For this review, take the finished solid that the model builds, in its own axes (mm). Face numbers are marked on the shaded views. A direction names the side the tool comes from. Coordinates: 2 decimals unless noted, no trailing zeros. Write each loop counter-clockwise with the first axis right and the second up, starting at its lowest first coordinate (ties: lowest second). Pieces come first, ordered by that corner, then holes. Notation, with made-up numbers: M 73.5,-1 L 87.5,-1 A27 ccw 87.5,26 Z; hole C 42,25 d10. An arc over 180 degrees is marked long. One line per question, with ' | ' between items.
from build123d import *

# Parameters (mm, degrees)
SKETCH1_R           = 6.35
BOSS_EXTRUDE1_DEPTH = 25.4
SKETCH2_W           = 26.416
SKETCH2_H           = 39.116
CUT_EXTRUDE1_DEPTH  = 26.4
SKETCH3_R           = 3.683
CUT_EXTRUDE2_DEPTH  = 6.842


with BuildPart() as part:
    # Sketch1 → Boss-Extrude1 (new body)
    with BuildSketch(Plane.XY):
        with BuildLine():
            Line((-50.8, 12.7), (50.8, 12.7))
            ThreePointArc((50.8, 12.7), (63.5, 0), (50.8, -12.7))
            Line((50.8, -12.7), (-50.8, -12.7))
            ThreePointArc((-50.8, -12.7), (-63.5, 0), (-50.8, 12.7))
        make_face()
        with Locations((-50.8, 0)):
            Circle(SKETCH1_R, mode=Mode.SUBTRACT)
        with Locations((50.8, 0)):
            Circle(SKETCH1_R, mode=Mode.SUBTRACT)
    extrude(amount=BOSS_EXTRUDE1_DEPTH)

    # Sketch2 → Cut-Extrude1 (cut, through all)
    with BuildSketch(Plane(origin=(0, 12.7, 0), x_dir=(1, 0, 0), z_dir=(0, 1, 0))):
        with Locations((0, -25.4)):
            Rectangle(SKETCH2_W, SKETCH2_H)
    extrude(amount=-CUT_EXTRUDE1_DEPTH, mode=Mode.SUBTRACT)

    # Sketch3 → Cut-Extrude2 (cut, through all)
    with BuildSketch(Plane.XY.offset(5.842)):
        Circle(SKETCH3_R)
    extrude(amount=-CUT_EXTRUDE2_DEPTH, mode=Mode.SUBTRACT)


solid = part.part
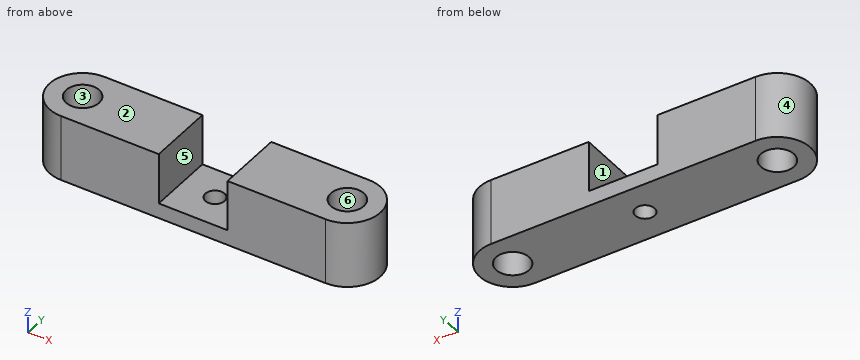
1) We need section C-C on x = 0. State the section outline as (y, z) points, then the cut area to 3 significant figures.
Responses:
outline: M -12.7,0 L -3.68,0 L -3.68,5.84 L -12.7,5.84 Z; M 3.68,0 L 12.7,0 L 12.7,5.84 L 3.68,5.84 Z | area: 105 mm^2
2) We need section D-D on y = -5. State the section outline as (x, z) points.
Responses:
outline: M -62.47,0 L -54.71,0 L -54.71,25.4 L -62.47,25.4 Z; M -46.89,0 L 46.89,0 L 46.89,25.4 L 13.21,25.4 L 13.21,5.84 L -13.21,5.84 L -13.21,25.4 L -46.89,25.4 Z; M 54.71,0 L 62.47,0 L 62.47,25.4 L 54.71,25.4 Z
3) To check wall thickness, follow line 1 along Y through (x, z) = (0, 2.75); line 2 along Y through (x, z) = (50.8, 16); line 3 along X through (y, z) = (-3, 24). State the ranges of each line that lie inside material, in increasing order. Write a range as [from, to].
Responses:
line 1: [-12.7, -3.68], [3.68, 12.7] | line 2: [-12.7, -6.35], [6.35, 12.7] | line 3: [-63.14, -56.4], [-45.2, -13.21], [13.21, 45.2], [56.4, 63.14]
4) We need section A-A on z = 11.75. State the section outline as (x, y) points.
Responses:
outline: M -50.8,-12.7 L -13.21,-12.7 L -13.21,12.7 L -50.8,12.7 A12.7 ccw Z; M 13.21,-12.7 L 50.8,-12.7 A12.7 ccw 50.8,12.7 L 13.21,12.7 Z; hole C -50.8,0 d12.7; hole C 50.8,0 d12.7
5) The part is to be moulded in two halves that separate along Y. For the marked faces 3, 4, 5 and 6, say which applies: +Y half, -Y half, draft (parallel to the pull), parting line (faces both ways), or undercut.
Responses:
face 3: undercut | face 4: parting line | face 5: draft | face 6: undercut
6) Insertion check: pin 1 Ø1.5 at (y, z) = (7.5, 17.5) entering from -X; pin 2 Ø4.5 at (x, y) = (0, 0) entering from +Z; pin 3 Ø1.5 at (y, z) = (9.5, 20.5) entering from +X. Each pin has a flat end and moves straight along its axis. Give the tip position at first contact, or say it passes through.
Responses:
pin 1: x = -61.56 | pin 2: through | pin 3: x = 60
7) Machinability: for the marked faces 1 and 2, which of the approach directions +Z, -Z, +X, -X, +Y, -Y give a long, thin tool a straight path to every point of the face, cutting with its end or side? Answer none if there is none.
Responses:
face 1: +Z, +Y, -Y | face 2: +Z, +X, -X, +Y, -Y
8) We need section B-B on y = 0. State the section outline as (x, z) points, then the cut area to 3 significant figures.
Responses:
outline: M -63.5,0 L -57.15,0 L -57.15,25.4 L -63.5,25.4 Z; M -44.45,0 L -3.68,0 L -3.68,5.84 L -13.21,5.84 L -13.21,25.4 L -44.45,25.4 Z; M 3.68,0 L 44.45,0 L 44.45,25.4 L 13.21,25.4 L 13.21,5.84 L 3.68,5.84 Z; M 57.15,0 L 63.5,0 L 63.5,25.4 L 57.15,25.4 Z | area: 2,020 mm^2
